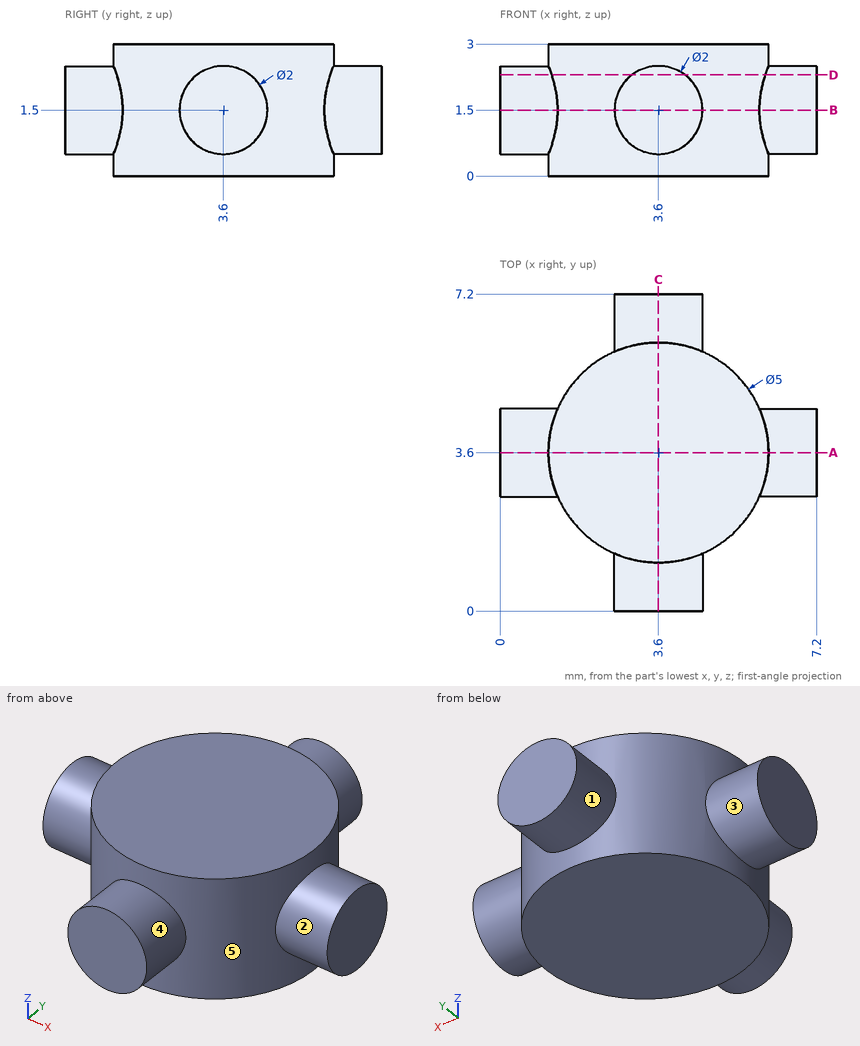
Geometry: see drawing. Coordinates: mm, zero at the bounding-box minimum. A direction names the side the tool comes from. Round coordinates to 2 decimals unless told otherwise and drop trailing zeros. Loops run counter-clockwise (first coordinate to the right, second up) from the corner with the lowest first, then second, coordinate; pieces in that order, holes last. Notation, with made-up numbers: (-31.5, -27.75) - (-12.5, -27.75) arc R21 ccw to (-12.5, -8.75) - close; hole circle Ø1 at (59, -9). An arc over 180 degrees is marked (long way). One line per item, written item: value. Start each with the question number.
(1) Access query for the marked faces 1, 2, 3, 4 and 5. Directions: +Z, -Z, +X, -X, +Y, -Y. A direction counts if a zero-diameter tool reaches every point of the face in a straight line with its end or side. Return the directions, or none.
(2) Section A-A, the plane y = 3.6. Return loops of the section in (x, z).
(3) Section B-B, the plane z = 1.5. Return loops of the section in (x, y), plus the area to 3 significant figures.
(4) Contact query for a flat-ended pin moving along its axis: P1, Ø1.5, axis at x = 3.5, y = 1, coming from the -Z side. Output: stop coordinate, or through.
(5) Ray query, line 1 (Y direction, x = 3.5, z = 2.85); line 2 (X direction, y = 6, z = 1.7). Return the intervals inside material, ascending. Write a range as [from, to].
(6) Section D-D, the plane z = 2.3. Return loops of the section in (x, y), plus the area to 3 significant figures.
Results below:
1. face 1: +Y
1. face 2: +X
1. face 3: -X
1. face 4: -Y
1. face 5: none
2. outline: (0, 0.5) - (1.1, 0.5) - (1.1, 0) - (6.1, 0) - (6.1, 0.5) - (7.2, 0.5) - (7.2, 2.5) - (6.1, 2.5) - (6.1, 3) - (1.1, 3) - (1.1, 2.5) - (0, 2.5) - close
3. outline: (0, 2.6) - (1.31, 2.6) arc R2.5 ccw to (2.6, 1.31) - (2.6, 0) - (4.6, 0) - (4.6, 1.31) arc R2.5 ccw to (5.89, 2.6) - (7.2, 2.6) - (7.2, 4.6) - (5.89, 4.6) arc R2.5 ccw to (4.6, 5.89) - (4.6, 7.2) - (2.6, 7.2) - (2.6, 5.89) arc R2.5 ccw to (1.31, 4.6) - (0, 4.6) - close
3. area: 29.0 mm^2
4. P1: z = 0
5. line 1: [1.1, 6.1]
5. line 2: [2.62, 4.58]
6. outline: (0, 3) - (1.17, 3) arc R2.5 ccw to (3, 1.17) - (3, 0) - (4.2, 0) - (4.2, 1.17) arc R2.5 ccw to (6.03, 3) - (7.2, 3) - (7.2, 4.2) - (6.03, 4.2) arc R2.5 ccw to (4.2, 6.03) - (4.2, 7.2) - (3, 7.2) - (3, 6.03) arc R2.5 ccw to (1.17, 4.2) - (0, 4.2) - close
6. area: 25.0 mm^2
